Geometry: final body of the model. Coordinates: model frame, mm. A direction names the side the tool comes from. Coordinates: 2 decimals unless noted, no trailing zeros. Write each loop counter-clockwise with the first axis right and the second up, starting at its lowest first coordinate (ties: lowest second). Pieces come first, ordered by that corner, then holes.
from build123d import *

# Parameters (mm, degrees)
SKETCH1_R           = 6.365
BOSS_EXTRUDE2_DEPTH = 7
CUT_EXTRUDE1_DEPTH  = 7
CIRPATTERN1_COUNT   = 20
SKETCH3_R           = 7.5
BOSS_EXTRUDE3_DEPTH = 2
FILLET1_R           = 2
BOSS_EXTRUDE4_START = 2
SKETCH4_R           = 7.5
BOSS_EXTRUDE4_DEPTH = 2
FILLET2_R           = 2
SKETCH5_R           = 4
CUT_EXTRUDE2_DEPTH  = 16.280706888


with BuildPart() as part:
    # Sketch1 → Boss-Extrude2 (new body)
    with BuildSketch(Plane(origin=(0, 0, 0), x_dir=(1, 0, 0), z_dir=(0, 1, 0))):
        with Locations(Location((0, 0, 0), (0, 0, 270))):
            Circle(SKETCH1_R)
    extrude(amount=BOSS_EXTRUDE2_DEPTH)

    # Sketch2 → Cut-Extrude1 (cut)
    with BuildSketch(Plane(origin=(0, 7, 0), x_dir=(1, 0, 0), z_dir=(0, 1, 0))):
        with BuildLine():
            Line((0, 5.985), (0.21554971, 5.985))
            ThreePointArc((0.21554971, 5.985), (0.330433243, 5.931445705), (0.363283354, 5.809023654))
            ThreePointArc((0.363283354, 5.809023654), (0.818934424, 5.170548463), (1.449584029, 5.636970529))
            ThreePointArc((1.449584029, 5.636970529), (1.518656835, 5.743249576), (1.644466755, 5.758681774))
            Line((1.644466755, 5.758681774), (1.849466711, 5.69207325))
            Line((1.849466711, 5.69207325), (1.966893169, 6.053474726))
            Line((1.966893169, 6.053474726), (1.188040248, 6.306539381))
            Line((1.188040248, 6.306539381), (0.818934424, 6.365))
            Line((0.818934424, 6.365), (0, 6.365))
            Line((0, 6.365), (0, 5.985))
        make_face()
    cut_extrude1 = extrude(amount=-CUT_EXTRUDE1_DEPTH, mode=Mode.SUBTRACT)

    # CirPattern1: Cut-Extrude1 ×20 about axis
    cirpattern1_axis = Axis((0, 0, 0), (0, 1, 0))
    for i in range(1, CIRPATTERN1_COUNT):
        add(cut_extrude1.rotate(cirpattern1_axis, i * 360 / CIRPATTERN1_COUNT), mode=Mode.SUBTRACT)

    # Sketch3 → Boss-Extrude3 (add)
    with BuildSketch(Plane(origin=(0, 7, 0), x_dir=(1, 0, 0), z_dir=(0, 1, 0))):
        with Locations(Location((0, 0, 0), (0, 0, 270))):
            Circle(SKETCH3_R)
    extrude(amount=BOSS_EXTRUDE3_DEPTH)

    # Fillet1
    fillet1_edges = [part.edges().sort_by_distance(p)[0] for p in [
        (0, 9, -7.5),
    ]]
    fillet(fillet1_edges, radius=FILLET1_R - 0.0001)  # a hair under: the kernel refuses the full size

    # Sketch4 → Boss-Extrude4 (add)
    with BuildSketch(Plane.XZ.offset(BOSS_EXTRUDE4_START)):
        with Locations(Location((0, 0, 0), (0, 0, 270))):
            Circle(SKETCH4_R)
    extrude(amount=-BOSS_EXTRUDE4_DEPTH)

    # Fillet2
    fillet2_edges = [part.edges().sort_by_distance(p)[0] for p in [
        (0, -2, 7.5),
    ]]
    fillet(fillet2_edges, radius=FILLET2_R - 0.0001)  # a hair under: the kernel refuses the full size

    # Sketch5 → Cut-Extrude2 (cut, through all)
    with BuildSketch(Plane.XZ.offset(2)):
        with Locations(Location((0, 0, 0), (0, 0, 270))):
            Circle(SKETCH5_R)
    extrude(amount=-CUT_EXTRUDE2_DEPTH, mode=Mode.SUBTRACT)


solid = part.part
Item 1: Material intervals for probe 1 along Z at (x, y) = (5.25, 1.75); probe 2 along Z at (x, y) = (-5.5, 1); probe 3 along X at (y, z) = (7.25, 0), sorted ascending.
Derived:
probe 1: z = -2.08 to -1.2, -0.61 to 0.61, 1.2 to 2.08
probe 2: z = -2.16 to -1.41, -0.4 to 0.4, 1.41 to 2.16
probe 3: x = -7.48 to -4, 4 to 7.48
Item 2: Pin query (flat end, axial travel): pin 1 (6 mm diameter, centred on x = -5.5, y = -1, fed in from -Z); pin 2 (3 mm diameter, centred on y = 2, z = 0.5, fed in from +X) (3 decimals); pin 3 (1 mm diameter, centred on x = 2.5, y = 3, fed in from +Z). Return the tip coordinate at first contact, or that it passes through.
Derived:
pin 1: stops at z = -7.02
pin 2: stops at x = 5.985
pin 3: stops at z = 5.64
Item 3: Set-up query: faces 3 (the cylindrical face through (-3.905, 3.423, 0.867)), 4 (the cylindrical face through (-4.66, 3.55, 2.39)). Return all of +Z, -Z, +X, -X, +Y, -Y with unobstructed straight access to the full face (end or side cutting, diameter ignored); none if empty.
Derived:
face 3: +Y, -Y
face 4: none
Item 4: Section A-A, the plane y = 8. Output: boundary loops of the cut face in (x, z), plus the area to 3 significant figures.
Derived:
outline: circle Ø14.46 at (0, 0); hole circle Ø8 at (0, 0)
area: 114 mm2
Item 5: Pull-direction query (X, two-part tool) for faces 1 (the flat face through (-2, 9, -4)), 2 (the cylindrical face through (-4.67, 3.55, -2.37)); classes: released by +X, released by -X, zero draft, split by the parting line, or undercut.
Derived:
face 1: zero draft
face 2: undercut
